from build123d import *

# Parameters (mm, degrees)
F1_DEPTH = 12.7
F2_T     = -1.27
F3_R     = 2.067279
F4_DEPTH = 6.35
F5_R     = 2.067279
F6_DEPTH = 6.35


with BuildPart() as f1:
    # F0 (on Top) → F1 (new body)
    with BuildSketch(Plane.XY):
        with BuildLine():
            Line((18.591051, 0), (6.35, 0))
            ThreePointArc((6.35, 0), (1.859872, -1.859872), (0, -6.35))
            Line((0, -6.35), (0, -33.910388))
            Line((0, -33.910388), (24.941051, -33.910388))
            Line((24.941051, -33.910388), (24.941051, -6.35))
            ThreePointArc((24.941051, -6.35), (23.081179, -1.859872), (18.591051, 0))
        make_face()
    extrude(amount=F1_DEPTH)

    # F2
    f2_openings = [f1.faces().sort_by_distance(p)[0] for p in [
        (12.470526, -17.279761, 12.7),
    ]]
    offset(amount=F2_T, openings=f2_openings)

    # F3 (on face) → F4 (join)
    with BuildSketch(Plane.XY.offset(1.27)):
        with Locations((4.631324, -5.627174)):
            Circle(F3_R)
    extrude(amount=F4_DEPTH)

    # F5 (on face) → F6 (join)
    with BuildSketch(Plane.XY.offset(1.27)):
        with Locations((4.949421, -28.45392)):
            Circle(F5_R)
        with Locations((20.426176, -5.810678)):
            Circle(F5_R)
        with Locations((20.982977, -28.639521)):
            Circle(F5_R)
    extrude(amount=F6_DEPTH)


solid = f1.part
The listing builds one solid part. Answer for the finished solid, in the listing's coordinates (mm). A direction names the side the tool comes from. Give positions to 0.01 mm unless a question says otherwise; leave off trailing zeros. Write each loop counter-clockwise with the first axis right and the second up, starting at its lowest first coordinate (ties: lowest second). Pieces come first, ordered by that corner, then holes.
Item 1: Section C-C, the plane z = 8.75 is taken. Write down the section's boundary in (x, y), plus the area to 3 significant figures.
Item 2: Determine the mould class of faces 1 (the cylindrical face through (1.91, -1.81, 6.26)), 2 (the cylindrical face through (18.36, -5.72, 4.4)), 3 (the flat face through (1.27, -19, 7)), 4 (the flat face through (24.941, -20, 6)) for opening direction X: released by +X, released by -X, zero draft, split by the parting line, or undercut.
Item 3: Section D-D, the plane y = -27 is taken. Write down the section's boundary in (x, z), plus the area to 3 significant figures.
Item 4: Find the intervals of material crossed by line 1 along X through (y, z) = (-27, 10.25); line 2 along X through (y, z) = (-30, 2.5); line 3 along Y through (x, z) = (6.5, 6), in increasing order.
Item 5: Which of the six approach directions +Z, -Z, +X, -X, +Y, -Y give full straight-line access (tool end or side, diameter ignored) to faces 5 (the flat face through (23.671, -20, 7)), 6 (the cylindrical face through (23.13, -1.91, 6.26))?
Item 6: Section A-A, the plane z = 4 is taken. Write down the section's boundary in (x, y), plus the area to 3 significant figures.
Item 7: Section B-B, the plane x = 11 is taken. Write down the section's boundary in (y, z).
Item 8: Flat-ended cylindrical pins translate along their axes: P1, Ø1.2, axis at x = 6, y = -28.5, coming from the +Z side; P2, Ø2, axis at x = 11, y = -23, coming from the +Z side. Find the tip coordinate at first contact, or state that the pin passes through.
Completed:
1. outline: (0, -33.91) - (24.94, -33.91) - (24.94, -6.35) arc R6.35 ccw to (18.59, 0) - (6.35, 0) arc R6.35 ccw to (0, -6.35) - close; hole (1.27, -32.64) - (23.67, -32.64) - (23.67, -6.35) arc R5.08 ccw to (18.59, -1.27) - (6.35, -1.27) arc R5.08 ccw to (1.27, -6.35) - close
1. area: 137 mm2
2. face 1: released by -X
2. face 2: undercut
2. face 3: undercut
2. face 4: released by +X
3. outline: (0, 0) - (24.94, 0) - (24.94, 12.7) - (23.67, 12.7) - (23.67, 1.27) - (22.24, 1.27) - (22.24, 7.62) - (19.72, 7.62) - (19.72, 1.27) - (6.42, 1.27) - (6.42, 7.62) - (3.48, 7.62) - (3.48, 1.27) - (1.27, 1.27) - (1.27, 12.7) - (0, 12.7) - close
3. area: 95.4 mm2
4. line 1: x = 0 to 1.27, 23.67 to 24.94
4. line 2: x = 0 to 1.27, 3.58 to 6.32, 19.43 to 22.54, 23.67 to 24.94
4. line 3: y = -33.91 to -32.64, -29.82 to -27.09, -6.51 to -4.74, -1.27 to 0
5. face 5: +Z
5. face 6: +Z, -Z, +X, +Y
6. outline: (0, -33.91) - (24.94, -33.91) - (24.94, -6.35) arc R6.35 ccw to (18.59, 0) - (6.35, 0) arc R6.35 ccw to (0, -6.35) - close; circle Ø4.13 at (4.63, -5.63); circle Ø4.13 at (4.95, -28.45); circle Ø4.13 at (20.43, -5.81); circle Ø4.13 at (20.98, -28.64); hole (1.27, -32.64) - (23.67, -32.64) - (23.67, -6.35) arc R5.08 ccw to (18.59, -1.27) - (6.35, -1.27) arc R5.08 ccw to (1.27, -6.35) - close
6. area: 191 mm2
7. outline: (-33.91, 0) - (0, 0) - (0, 12.7) - (-1.27, 12.7) - (-1.27, 1.27) - (-32.64, 1.27) - (-32.64, 12.7) - (-33.91, 12.7) - close
8. P1: stops at z = 7.62
8. P2: stops at z = 1.27
